Here's how the part is built. I have some questions about the finished solid (model axes, mm). A direction names the side the tool comes from. Coordinates: 2 decimals unless noted, no trailing zeros. Write each loop counter-clockwise with the first axis right and the second up, starting at its lowest first coordinate (ties: lowest second). Pieces come first, ordered by that corner, then holes.
(1) Thinking about a two-plate mould opening in X: for faces 5 (the flat face through (34, 51, -2.54)), 6 (the flat face through (64.77, 3, -1)), 7 (the flat face through (68.268, 39.488, -0.036)), which applies, released by +X, released by -X, zero draft, split by the parting line, or undercut?
(2) Imagine slicing it at C-C, the plane x = 35.5. List the corners of the cut face in (y, z) for me, plus the area to 3 significant figures.
(3) Which directions (+Z, -Z, +X, -X, +Y, -Y) give clear straight access to the entire face, cutting with the end or side of a thin tool? Please do faces 1 (the flat face through (66.98, 1, 0)), 2 (the flat face through (38, 4.14, -1)), 3 (the flat face through (45, 3.334, -1)), 4 (the flat face through (66.98, 46, 0)).
(4) Imagine slicing it at B-B, the plane z = 1.65. List the corners of the cut face in (x, y) for me.
(5) Please list where these lines run through material, in increasing order: probe 1 along Y at (x, z) = (26, -1.2); probe 2 along Y at (x, z) = (23, -1.05); probe 3 along Y at (x, z) = (22, 2.25).
(6) Imagine slicing it at A-A, the plane y = 11. List the corners of the cut face in (x, z) for me, plus the area to 3 significant figures.
(7) For pin 1 Ø16 at (x, y) = (37.5, 17.5) entering from +Z; pin 2 Ø1.3 at (y, z) = (3, -1) entering from +X; pin 3 Ø0.6 at (x, y) = (-0.5, 8.5) entering from +Z; pin 4 Ø1.5 at (y, z) = (47.5, 0) entering from +X, each with a flat end and sliding along its axis, tell me the tip position at first contact or that it passes through.
(8) Imagine slicing it at D-D, the plane x = 13. List the corners of the cut face in (y, z) for me.
Autodesk Inventor part; units mm, degrees
ref_plane "YZ Plane" through (0, 0, 0) normal (1, 0, 0) x (0, 1, 0)
ref_plane "XZ Plane" through (0, 0, 0) normal (0, 1, 0) x (-1, 0, 0)
ref_plane "XY Plane" through (0, 0, 0) normal (0, 0, 1) x (1, 0, 0)
sketch "Sketch1" plane through (0, 0, 0) normal (0, 0, 1) x (1, 0, 0)
  line L0 (0, 53.34) -> (64.516, 53.34)
  line L1 (64.516, 53.34) -> (66.04, 51.816)
  line L2 (66.04, 51.816) -> (66.04, 40.386)
  line L3 (66.04, 40.386) -> (68.58, 37.846)
  line L4 (68.58, 37.846) -> (68.58, 5.08)
  line L5 (66.04, 0) -> (0, 0)
  line L6 (0, 0) -> (0, 53.34)
  line L7 (68.58, 5.08) -> (66.04, 2.54)
  line L8 (66.04, 2.54) -> (66.04, 0)
  line L9 (64.9053, 54.2798) -> (-0.9398, 54.2798)
  line L10 (-0.9398, 54.2798) -> (-0.9398, -0.9398)
  line L11 (-0.9398, -0.9398) -> (66.9798, -0.9398)
  line L12 (66.9798, -0.9398) -> (66.9798, 2.1507)
  line L13 (66.9798, 2.1507) -> (69.5198, 4.6907)
  line L14 (69.5198, 4.6907) -> (69.5198, 38.2353)
  line L15 (69.5198, 38.2353) -> (66.9798, 40.7753)
  line L16 (66.9798, 40.7753) -> (66.9798, 52.2053)
  line L17 (66.9798, 52.2053) -> (64.9053, 54.2798)
  line L18 (64.6002, 53.5432) -> (-0.2032, 53.5432)
  line L19 (-0.2032, 53.5432) -> (-0.2032, -0.2032)
  line L20 (-0.2032, -0.2032) -> (66.2432, -0.2032)
  line L21 (66.2432, -0.2032) -> (66.2432, 2.4558)
  line L22 (66.2432, 2.4558) -> (68.7832, 4.9958)
  line L23 (68.7832, 4.9958) -> (68.7832, 37.9302)
  line L24 (68.7832, 37.9302) -> (66.2432, 40.4702)
  line L25 (66.2432, 40.4702) -> (66.2432, 51.9002)
  line L26 (66.2432, 51.9002) -> (64.6002, 53.5432)
  point P0 (0, 0)
  dimension "d0" = 64.516
  dimension "d1" = 53.34
  dimension "d4" = 66.04
  dimension "d5" = 51.816
  dimension "d6" = 68.58
  dimension "d7" = 40.386
  dimension "d8" = 37.846
  dimension "d9" = 66.04
  dimension "d10" = 2.54
  dimension "d11" = 5.08
  dimension "d15" = 0.2032
  dimension "d18" = 0.7366
extrude "Extrusion2" add sketch "Sketch1" along normal blind 2.54 contours L17 L16 L15 L14 L13 L12 L11 L10 L9
sketch "Sketch2" plane through (0, 0, 0) normal (0, 0, 1) x (1, 0, 0)
  line L0 (0, 53.34) -> (64.516, 53.34)
  line L1 (64.516, 53.34) -> (66.04, 51.816)
  line L2 (66.04, 51.816) -> (66.04, 40.386)
  line L3 (66.04, 40.386) -> (68.58, 37.846)
  line L4 (68.58, 37.846) -> (68.58, 5.08)
  line L5 (66.04, 0) -> (0, 0)
  line L6 (0, 0) -> (0, 53.34)
  line L7 (68.58, 5.08) -> (66.04, 2.54)
  line L8 (66.04, 2.54) -> (66.04, 0)
  line L9 (64.9053, 54.2798) -> (-0.9398, 54.2798)
  line L10 (-0.9398, 54.2798) -> (-0.9398, -0.9398)
  line L11 (-0.9398, -0.9398) -> (66.9798, -0.9398)
  line L12 (66.9798, -0.9398) -> (66.9798, 2.1507)
  line L13 (66.9798, 2.1507) -> (69.5198, 4.6907)
  line L14 (69.5198, 4.6907) -> (69.5198, 38.2353)
  line L15 (69.5198, 38.2353) -> (66.9798, 40.7753)
  line L16 (66.9798, 40.7753) -> (66.9798, 52.2053)
  line L17 (66.9798, 52.2053) -> (64.9053, 54.2798)
  line L18 (64.6002, 53.5432) -> (-0.2032, 53.5432)
  line L19 (-0.2032, 53.5432) -> (-0.2032, -0.2032)
  line L20 (-0.2032, -0.2032) -> (66.2432, -0.2032)
  line L21 (66.2432, -0.2032) -> (66.2432, 2.4558)
  line L22 (66.2432, 2.4558) -> (68.7832, 4.9958)
  line L23 (68.7832, 4.9958) -> (68.7832, 37.9302)
  line L24 (68.7832, 37.9302) -> (66.2432, 40.4702)
  line L25 (66.2432, 40.4702) -> (66.2432, 51.9002)
  line L26 (66.2432, 51.9002) -> (64.6002, 53.5432)
  line L27 (4.1402, 49.1998) -> (61.8998, 49.1998)
  line L28 (61.8998, 49.1998) -> (61.8998, 38.6711)
  line L29 (61.8998, 38.6711) -> (64.4398, 36.1311)
  line L30 (64.4398, 6.7949) -> (61.8998, 4.2549)
  line L31 (61.8998, 4.2549) -> (61.8998, 4.1402)
  line L32 (61.8998, 4.1402) -> (4.1402, 4.1402)
  line L33 (4.1402, 4.1402) -> (4.1402, 49.1998)
  line L34 (63.627, 30.43) -> (66.167, 30.43) construction
  line L35 (66.167, 30.43) -> (66.167, 25.35) construction
  line L36 (66.167, 25.35) -> (63.627, 25.35) construction
  line L37 (63.627, 25.35) -> (63.627, 30.43) construction
  line L38 (64.4398, 36.1311) -> (64.4398, 0)
  circle A0 centre (15.24, 50.8) radius 1.5875
  circle A1 centre (66.04, 35.3568) radius 1.5875
  circle A2 centre (65.8368, 7.62) radius 1.5875
  circle A3 centre (13.97, 2.54) radius 1.5875
  point P0 (0, 0)
  point P1 (0, 1.4137)
  dimension "d19" = 64.516
  dimension "d20" = 53.34
  dimension "d21" = 66.04
  dimension "d22" = 51.816
  dimension "d23" = 68.58
  dimension "d24" = 40.386
  dimension "d25" = 37.846
  dimension "d26" = 66.04
  dimension "d27" = 2.54
  dimension "d28" = 5.08
  dimension "d29" = 0.2032
  dimension "d30" = 0.7366
  dimension "d31" = 5.08
  dimension "d56" = 30.43
  dimension "d57" = 63.627
  dimension "d58" = 5.08
  dimension "d61" = 2.54
  dimension "d70" = 13.97
  dimension "d71" = 2.54
  dimension "d72" = 3.175
  dimension "d73" = 50.8
  dimension "d74" = 3.175
  dimension "d75" = 15.24
  dimension "d76" = 66.04
  dimension "d77" = 35.56
  dimension "d78" = 3.175
  dimension "d79" = 3.175
  dimension "d80" = 66.04
  dimension "d81" = 7.62
extrude "Extrusion3" add sketch "Sketch2" against normal blind 2.54 contours L0 L1 L2 L3 L4 L7 L8 L5 L6 | A2 L38 | L38 A2 | L17 L16 L15 L14 L13 L12 L11 L10 L9 | L26 L25 L24 L23 L22 L21 L20 L19 L18 | A0 | A1 | A3
sketch "Sketch4" plane through (0, 0, 2.54) normal (0, 0, 1) x (1, 0, 0)
  line L0 (-0.2032, -0.2032) -> (-0.2032, 53.5432)
  line L1 (-0.9398, -0.9398) -> (-0.9398, 54.2798)
  line L2 (-0.2032, 12.446) -> (-0.9398, 12.446)
  line L3 (-0.2032, 2.8575) -> (-0.9398, 2.8575)
  line L4 (-0.2032, 32.004) -> (-0.9398, 32.004)
  line L5 (-0.2032, 44.196) -> (-0.9398, 44.196)
  point P0 (0, 0)
  dimension "d35" = 12.446
  dimension "d36" = 2.8575
  dimension "d37" = 32.004
  dimension "d38" = 44.196
extrude "Extrusion4" cut sketch "Sketch4" against normal blind 2.286 contours L3 L1 L2 L0 | L4 L1 L5 L0
sketch "Sketch5" plane through (0, 0, 0) normal (0, 0, 1) x (1, 0, 0)
  line L0 (25.4, 3.3338) -> (64.77, 3.3338)
  line L1 (64.77, 3.3338) -> (64.77, 1.7463)
  line L2 (64.77, 1.7463) -> (25.4, 1.7463)
  line L3 (25.4, 1.7463) -> (25.4, 3.3338)
  line L4 (17.78, 51.5938) -> (64.77, 51.5938)
  line L5 (64.77, 51.5938) -> (64.77, 50.0062)
  line L6 (64.77, 50.0062) -> (17.78, 50.0062)
  line L7 (17.78, 50.0062) -> (17.78, 51.5938)
  line L8 (-0.2032, 53.5432) -> (-0.2032, -0.2032)
  line L9 (-0.2032, 12.065) -> (11.2268, 12.065)
  line L10 (11.2268, 12.065) -> (11.2268, 1.6002)
  line L11 (11.2268, 1.6002) -> (-0.2032, 1.6002)
  line L12 (-0.2032, 1.6002) -> (-0.2032, 12.065)
  line L13 (1.6002, 12.065) -> (1.6002, 1.6002)
  line L14 (63.627, 30.43) -> (66.167, 30.43) construction
  line L15 (63.627, 25.35) -> (63.627, 30.43) construction
  line L16 (66.167, 30.43) -> (66.167, 25.35) construction
  line L17 (66.167, 25.35) -> (63.627, 25.35) construction
  line L18 (4.1402, 4.1402) -> (4.1402, 49.1998)
  line L19 (4.1402, 49.1998) -> (61.8998, 49.1998)
  line L20 (61.8998, 49.1998) -> (61.8998, 38.6711)
  line L21 (61.8998, 38.6711) -> (64.4398, 36.1311)
  line L22 (64.4398, 6.866) -> (64.4398, 6.7949)
  line L23 (64.4398, 6.7949) -> (61.8998, 4.2549)
  line L24 (61.8998, 4.2549) -> (61.8998, 4.1402)
  line L25 (61.8998, 4.1402) -> (4.1402, 4.1402)
  line L26 (66.2432, 51.9002) -> (64.6002, 53.5432)
  line L27 (64.6002, 53.5432) -> (-0.2032, 53.5432)
  line L28 (-0.2032, 53.5432) -> (-0.2032, -0.2032)
  line L29 (-0.2032, -0.2032) -> (66.2432, -0.2032)
  line L30 (66.2432, -0.2032) -> (66.2432, 2.4558)
  line L31 (66.2432, 2.4558) -> (68.7832, 4.9958)
  line L32 (68.7832, 4.9958) -> (68.7832, 37.9302)
  line L33 (68.7832, 37.9302) -> (66.2432, 40.4702)
  line L34 (66.2432, 40.4702) -> (66.2432, 51.9002)
  line L35 (64.4398, 36.1311) -> (64.4398, 6.7949)
  line L36 (64.4398, 33.732) -> (66.9798, 31.192)
  line L37 (64.4398, 22.048) -> (66.9798, 24.588)
  line L38 (66.9798, 31.192) -> (66.9798, 24.588)
  line L39 (64.4398, 33.732) -> (64.4398, 22.048)
  line L40 (61.8998, 4.1402) -> (4.1402, 4.1402)
  line L41 (4.1402, 4.1402) -> (4.1402, 49.1998)
  line L42 (1.6002, 44.4853) -> (4.1402, 47.0253)
  line L43 (66.2432, 40.4702) -> (66.2432, 51.9002)
  line L44 (1.6002, 31.7147) -> (4.1402, 29.1747)
  line L45 (1.6002, 31.7147) -> (1.6002, 44.4853)
  line L46 (4.1402, 47.0253) -> (4.1402, 29.1747)
  arc A0 (64.4398, 8.374) -> (64.4398, 6.866) centre (65.8368, 7.62) ccw
  line L47 (64.4398, 36.1311) -> (64.4398, 8.374)
  point P0 (0, 0)
  point P1 (64.4398, 31.192)
  point P2 (64.4398, 31.192)
  point P3 (64.4398, 24.588)
  point P4 (64.4398, 24.588)
  dimension "d41" = 1.5875
  dimension "d42" = 25.4
  dimension "d43" = 64.77
  dimension "d44" = 17.78
  dimension "d45" = 64.77
  dimension "d46" = 1.5875
  dimension "d47" = 51.5938
  dimension "d48" = 1.7463
  dimension "d51" = 0
  dimension "d52" = 12.065
  dimension "d54" = 11.43
  dimension "d66" = 2.54
  dimension "d67" = 2.54
  dimension "d68" = 2.54
  dimension "d69" = 2.54
  dimension "d97" = 2.54
  dimension "d101" = 2.54
  dimension "d102" = 2.54
extrude "Extrusion5" cut sketch "Sketch5" against normal blind 2.159 contours L0 L1 L2 L3 | L4 L5 L6 L7
sketch "Sketch7" plane through (0, 0, 0) normal (0, 0, 1) x (1, 0, 0)
  line L0 (25.4, 3.3338) -> (64.77, 3.3338)
  line L1 (64.77, 3.3338) -> (64.77, 1.7463)
  line L2 (64.77, 1.7463) -> (25.4, 1.7463)
  line L3 (25.4, 1.7463) -> (25.4, 3.3338)
  line L4 (17.78, 51.5938) -> (64.77, 51.5938)
  line L5 (64.77, 51.5938) -> (64.77, 50.0062)
  line L6 (64.77, 50.0062) -> (17.78, 50.0062)
  line L7 (17.78, 50.0062) -> (17.78, 51.5938)
  line L8 (-0.2032, 53.5432) -> (-0.2032, -0.2032)
  line L9 (-0.2032, 12.065) -> (11.2268, 12.065)
  line L10 (11.2268, 12.065) -> (11.2268, 1.6002)
  line L11 (11.2268, 1.6002) -> (-0.2032, 1.6002)
  line L12 (-0.2032, 1.6002) -> (-0.2032, 12.065)
  line L13 (1.6002, 12.065) -> (1.6002, 1.6002)
  line L14 (63.627, 30.43) -> (66.167, 30.43) construction
  line L15 (63.627, 25.35) -> (63.627, 30.43) construction
  line L16 (66.167, 30.43) -> (66.167, 25.35) construction
  line L17 (66.167, 25.35) -> (63.627, 25.35) construction
  line L18 (4.1402, 4.1402) -> (4.1402, 49.1998)
  line L19 (4.1402, 49.1998) -> (61.8998, 49.1998)
  line L20 (61.8998, 49.1998) -> (61.8998, 38.6711)
  line L21 (61.8998, 38.6711) -> (64.4398, 36.1311)
  line L22 (64.4398, 6.866) -> (64.4398, 6.7949)
  line L23 (64.4398, 6.7949) -> (61.8998, 4.2549)
  line L24 (61.8998, 4.2549) -> (61.8998, 4.1402)
  line L25 (61.8998, 4.1402) -> (4.1402, 4.1402)
  line L26 (66.2432, 51.9002) -> (64.6002, 53.5432)
  line L27 (64.6002, 53.5432) -> (-0.2032, 53.5432)
  line L28 (-0.2032, 53.5432) -> (-0.2032, -0.2032)
  line L29 (-0.2032, -0.2032) -> (66.2432, -0.2032)
  line L30 (66.2432, -0.2032) -> (66.2432, 2.4558)
  line L31 (66.2432, 2.4558) -> (68.7832, 4.9958)
  line L32 (68.7832, 4.9958) -> (68.7832, 37.9302)
  line L33 (68.7832, 37.9302) -> (66.2432, 40.4702)
  line L34 (66.2432, 40.4702) -> (66.2432, 51.9002)
  line L35 (64.4398, 36.1311) -> (64.4398, 6.7949)
  line L36 (64.4398, 33.732) -> (66.9798, 31.192)
  line L37 (64.4398, 22.048) -> (66.9798, 24.588)
  line L38 (66.9798, 31.192) -> (66.9798, 24.588)
  line L39 (64.4398, 33.732) -> (64.4398, 22.048)
  line L40 (61.8998, 4.1402) -> (4.1402, 4.1402)
  line L41 (4.1402, 4.1402) -> (4.1402, 49.1998)
  line L42 (1.6002, 44.4853) -> (4.1402, 47.0253)
  line L43 (66.2432, 40.4702) -> (66.2432, 51.9002)
  line L44 (1.6002, 31.7147) -> (4.1402, 29.1747)
  line L45 (1.6002, 31.7147) -> (1.6002, 44.4853)
  line L46 (4.1402, 47.0253) -> (4.1402, 29.1747)
  arc A0 (64.4398, 8.374) -> (64.4398, 6.866) centre (65.8368, 7.62) ccw
  line L47 (64.4398, 36.1311) -> (64.4398, 8.374)
  point P0 (0, 0)
  point P1 (0, 0)
  point P2 (64.4398, 31.192)
  point P3 (64.4398, 31.192)
  point P4 (64.4398, 24.588)
  point P5 (64.4398, 24.588)
  dimension "d106" = 1.5875
  dimension "d107" = 25.4
  dimension "d108" = 64.77
  dimension "d109" = 17.78
  dimension "d110" = 64.77
  dimension "d111" = 1.5875
  dimension "d112" = 51.5938
  dimension "d113" = 1.7463
  dimension "d114" = 0
  dimension "d115" = 12.065
  dimension "d116" = 11.43
  dimension "d117" = 2.54
  dimension "d118" = 2.54
  dimension "d119" = 2.54
  dimension "d120" = 2.54
  dimension "d121" = 2.54
  dimension "d122" = 2.54
  dimension "d123" = 2.54
extrude "Extrusion7" cut sketch "Sketch7" against normal through all contours L9 L18 L25 L10 L11 L13 | L9 L10 L25 L18 | L44 L45 L42 L18 | L36 L38 L37 L35
chamfer "Chamfer3" distance 2.54 angle 45 2 edges at (4.1402, 12.065, -1.27) (11.2268, 4.1402, -1.27)
chamfer "Chamfer5" distance 2.54 angle 45 1 edges at (1.6002, 1.6002, -1.27)
equation "\"d97\" = d101"
equation "\"d102\" = d101"
properties part number "Arduino Bumper 0005"
Recorded:
1. face 5: zero draft
1. face 6: undercut
1. face 7: released by +X
2. outline: (-0.94, -2.54) - (4.14, -2.54) - (4.14, 0) - (3.33, 0) - (3.33, -2.16) - (1.75, -2.16) - (1.75, 0) - (-0.2, 0) - (-0.2, 2.54) - (-0.94, 2.54) - close; (49.2, -2.54) - (54.28, -2.54) - (54.28, 2.54) - (53.54, 2.54) - (53.54, 0) - (51.59, 0) - (51.59, -2.16) - (50.01, -2.16) - (50.01, 0) - (49.2, 0) - close
2. area: 22.7 mm2
3. face 1: +Z, -Z, +X, -Y
3. face 2: +Z, -Z
3. face 3: +Z
3. face 4: +Z, -Z, +X, +Y
4. outline: (-0.94, -0.94) - (66.98, -0.94) - (66.98, 2.15) - (69.52, 4.69) - (69.52, 38.24) - (66.98, 40.78) - (66.98, 52.21) - (64.91, 54.28) - (-0.94, 54.28) - (-0.94, 44.2) - (-0.2, 44.2) - (-0.2, 53.54) - (64.6, 53.54) - (66.24, 51.9) - (66.24, 40.47) - (68.78, 37.93) - (68.78, 5) - (66.24, 2.46) - (66.24, -0.2) - (-0.2, -0.2) - (-0.2, 2.86) - (-0.94, 2.86) - close; (-0.94, 12.45) - (-0.2, 12.45) - (-0.2, 32) - (-0.94, 32) - close
5. probe 1: y = -0.94 to 1.75, 3.33 to 4.14, 49.2 to 50.01, 51.59 to 54.28
5. probe 2: y = -0.94 to 4.14, 49.2 to 50.01, 51.59 to 54.28
5. probe 3: y = -0.94 to -0.2, 53.54 to 54.28
6. outline: (-0.94, -2.54) - (1.6, -2.54) - (1.6, 0) - (-0.2, 0) - (-0.2, 0.25) - (-0.94, 0.25) - close; (64.44, -2.54) - (69.52, -2.54) - (69.52, 2.54) - (68.78, 2.54) - (68.78, 0) - (64.44, 0) - close
6. area: 21.4 mm2
7. pin 1: passes through
7. pin 2: stops at x = 68.48
7. pin 3: stops at z = 0.25
7. pin 4: stops at x = 66.98
8. outline: (-0.94, -2.54) - (3.37, -2.54) - (3.37, 0) - (-0.2, 0) - (-0.2, 2.54) - (-0.94, 2.54) - close; (49.2, -2.54) - (54.28, -2.54) - (54.28, 2.54) - (53.54, 2.54) - (53.54, 0) - (49.2, 0) - close
